Could you check a few things on this model? Use its own coordinates, in mm. A direction names the side the tool comes from. Coordinates: 2 decimals unless noted, no trailing zeros. Order: outer loops, then holes, each group sorted by start corner. A loop starts at its lowest first (then second) coordinate and runs counter-clockwise, first axis right, second up. Notation, with made-up numbers: (37.25, 74.5) -> (51.25, 74.5) arc R32 cw to (51.25, 109.5) -> close; hole circle Ø1 at (59.25, 60). An arc over 180 degrees is marked (long way). Use a Markdown table: item, result. Add a question column.
1) Will these pins go through, and if not, where does the flat tip stop? pin 1 Ø4 at (x, z) = (22.5, 7.5) entering from +Y; pin 2 Ø4 at (x, z) = (15, 1.5) entering from +Y; pin 3 Ø8 at (x, z) = (40, 5.5) entering from +Y.
2) If we section it at D-D (y = 79): Write out the boundary of the cut face in (x, z).
3) If we section it at C-C (z = 6.75): Give the number of separate pieces and of enclosed holes in the cut face, plus the area to 3 significant figures.
4) If we section it at B-B (y = 23): Write out the boundary of the cut face in (x, z).
5) If I drill on L1, parallel to X at y = 195.5, z = 7.75; L2, parallel to Y at x = 12, z = 9.5; L3, parallel to Y at x = 18.5, z = 2.75, over which ranges is the centre line in solid material (lowest first)? Write a range as [from, to].
6) If we section it at A-A (x = 30): Write out the boundary of the cut face in (y, z).
7) Which directions (+Z, -Z, +X, -X, +Y, -Y) give clear straight access to the entire face, cutting with the end or side of a thin tool? Please do faces 5 (the flat face through (50.4, 95, 15)), 6 (the flat face through (45, 161, 8)).
8) Thinking about a two-plate mould opening in Y: for faces 1 (the flat face through (30, 240, 7)), 2 (the cylindrical face through (10, 79, 8)), 3 (the flat face through (0, 106, 7)), 4 (the flat face through (30, 0, 7)), which applies, +Y half, -Y half, draft (parallel to the pull), parting line (faces both ways), or undercut?
```python
from build123d import *

# Parameters (mm, degrees)
BASE_EXTRUSION_DEPTH       = 15
ESQUISSE2_R                = 15
ENL_V_MAT_EXTRU_1_DEPTH    = 15
ENL_V_MAT_EXTRU_2_DEPTH    = 15
ESQUISSE4_R                = 4
ENL_V_MAT_EXTRU_3_DEPTH    = 248.840674628
ENL_V_MAT_EXTRU_4_DEPTH    = 248.840674658
R_P_TITION_LIN_AIRE1_COUNT = 2
R_P_TITION_LIN_AIRE1_PITCH = 94.21


with BuildPart() as part:
    # Esquisse1 → Base-Extrusion (new body)
    with BuildSketch(Plane.XY):
        Polygon((0, 215), (25, 240), (35, 240), (60, 215), (60, 0), (0, 0), align=None)
    extrude(amount=BASE_EXTRUSION_DEPTH)

    # Esquisse2 → Enlèv. mat.-Extru.1 (cut)
    with BuildSketch(Plane.XY.offset(15)):
        with Locations((30, 23)):
            Circle(ESQUISSE2_R)
    extrude(amount=-ENL_V_MAT_EXTRU_1_DEPTH, mode=Mode.SUBTRACT)

    # Esquisse3 → Enlèv. mat.-Extru.2 (cut)
    with BuildSketch(Plane.XY.offset(15)):
        with BuildLine():
            Line((45, 91), (45, 84))
            ThreePointArc((45, 84), (50, 79), (45, 74))
            Line((45, 74), (15, 74))
            ThreePointArc((15, 74), (10, 79), (15, 84))
            Line((15, 84), (15, 91))
            ThreePointArc((15, 91), (10, 96), (15, 101))
            Line((15, 101), (15, 220))
            ThreePointArc((15, 220), (30, 235), (45, 220))
            Line((45, 220), (45, 101))
            ThreePointArc((45, 101), (50, 96), (45, 91))
        make_face()
    extrude(amount=-ENL_V_MAT_EXTRU_2_DEPTH, mode=Mode.SUBTRACT)

    # Esquisse4 → Enlèv. mat.-Extru.3 (cut, through all)
    with BuildSketch(Plane.ZY):
        with Locations((7.5, 23)):
            Circle(ESQUISSE4_R)
    extrude(amount=-ENL_V_MAT_EXTRU_3_DEPTH, mode=Mode.SUBTRACT)

    # Esquisse5 → Enlèv. mat.-Extru.4 (cut, through all)
    with BuildSketch(Plane.XY.offset(15)):
        Polygon((14.902218658, 116.777944848), (12.23927057, 118.377944848), (12.23927057, 115.177944848), align=None)
    enl_v_mat_extru_4 = extrude(amount=-ENL_V_MAT_EXTRU_4_DEPTH, mode=Mode.SUBTRACT)

    # Répétition linéaire1: Enlèv. mat.-Extru.4 ×2
    with Locations(*[(0, i * R_P_TITION_LIN_AIRE1_PITCH, 0) for i in range(1, R_P_TITION_LIN_AIRE1_COUNT)]):
        add(enl_v_mat_extru_4, mode=Mode.SUBTRACT)


solid = part.part
```
Answer sheet:
| question | item | result |
|---|---|---|
| 1 | pin 1 | y = 239.5 |
| 1 | pin 2 | y = 232 |
| 1 | pin 3 | y = 239 |
| 2 | outline | (0, 0) -> (10, 0) -> (10, 15) -> (0, 15) -> close; (50, 0) -> (60, 0) -> (60, 15) -> (50, 15) -> close |
| 3 | separate pieces | 2 |
| 3 | enclosed holes | 3 |
| 3 | area | 7,930 mm2 |
| 4 | outline | (0, 0) -> (15, 0) -> (15, 3.5) -> (0, 3.5) -> close; (0, 11.5) -> (15, 11.5) -> (15, 15) -> (0, 15) -> close; (45, 0) -> (60, 0) -> (60, 3.5) -> (45, 3.5) -> close; (45, 11.5) -> (60, 11.5) -> (60, 15) -> (45, 15) -> close |
| 5 | L1 | [0, 15], [45, 60] |
| 5 | L2 | [0, 19.54], [26.46, 75], [83, 92], [100, 227] |
| 5 | L3 | [0, 13.37], [32.63, 74], [229.63, 233.5] |
| 6 | outline | (0, 0) -> (8, 0) -> (8, 15) -> (0, 15) -> close; (38, 0) -> (74, 0) -> (74, 15) -> (38, 15) -> close; (235, 0) -> (240, 0) -> (240, 15) -> (235, 15) -> close |
| 7 | face 5 | +Z, +X, -X, +Y, -Y |
| 7 | face 6 | +Z, -Z |
| 8 | face 1 | +Y half |
| 8 | face 2 | undercut |
| 8 | face 3 | draft |
| 8 | face 4 | -Y half |
